Read the model definition and answer for the solid it produces. Units are mm, in the model's axes. A direction names the side the tool comes from. Coordinates: 2 decimals unless noted, no trailing zeros. Loops run counter-clockwise (first coordinate to the right, second up) from the corner with the lowest first, then second, coordinate; pieces in that order, holes last.
from build123d import *

# Parameters (mm, degrees)
F1_DEPTH = 76.2
F2_DEPTH = 211.582
F3_R     = 6.35
F4_DEPTH = 296.926


with BuildPart() as f1:
    # F0 (on Front) → F1 (new body)
    with BuildSketch(Plane.XZ):
        with BuildLine():
            Line((-75.994186, -26.958708), (-75.994186, -65.058708))
            Line((-75.994186, -65.058708), (0.205814, -65.058708))
            Line((0.205814, -65.058708), (0.205814, -26.958708))
            Line((0.205814, -26.958708), (41.952003, 20.148002))
            ThreePointArc((41.952003, 20.148002), (37.907157, 19.552642), (36.629202, 23.436206))
            Line((36.629202, 23.436206), (-37.894186, -26.958708))
            Line((-37.894186, -26.958708), (-110.240799, 29.427088))
            ThreePointArc((-110.240799, 29.427088), (-109.339718, 28.31636), (-109.017566, 26.922845))
            ThreePointArc((-109.017566, 26.922845), (-110.631205, 24.158288), (-113.831913, 24.203807))
            Line((-113.831913, 24.203807), (-75.994186, -26.958708))
        make_face()
        with BuildLine():
            ThreePointArc((36.629202, 23.436206), (37.907157, 19.552642), (41.952003, 20.148002))
            ThreePointArc((41.952003, 20.148002), (42.544402, 21.127687), (42.750814, 22.253792))
            ThreePointArc((42.750814, 22.253792), (41.820878, 24.498856), (39.575814, 25.428792))
            Line((39.575814, 25.428792), (36.629202, 23.436206))
        make_face()
        with BuildLine():
            ThreePointArc((-110.240799, 29.427088), (-114.808874, 28.721611), (-113.831913, 24.203807))
            ThreePointArc((-113.831913, 24.203807), (-110.631205, 24.158288), (-109.017566, 26.922845))
            ThreePointArc((-109.017566, 26.922845), (-109.339718, 28.31636), (-110.240799, 29.427088))
        make_face()
    extrude(amount=F1_DEPTH)

    # F1_face (on face) → F2 (cut)
    with BuildSketch(Plane(origin=(-38.414118, 0, -27.709483), x_dir=(1, 0, 0), z_dir=(0, 1, 0))):
        with BuildLine():
            Line((-37.580068, 37.349226), (-37.580068, -0.750774))
            Line((-37.580068, -0.750774), (-75.417795, -51.91329))
            ThreePointArc((-75.417795, -51.91329), (-76.394756, -56.431093), (-71.826681, -57.13657))
            Line((-71.826681, -57.13657), (0.519932, -0.750774))
            Line((0.519932, -0.750774), (77.989932, -53.138274))
            ThreePointArc((77.989932, -53.138274), (80.234996, -52.208338), (81.164932, -49.963274))
            ThreePointArc((81.164932, -49.963274), (80.958519, -48.837169), (80.366121, -47.857484))
            Line((80.366121, -47.857484), (38.619932, -0.750774))
            Line((38.619932, -0.750774), (38.619932, 37.349226))
            Line((38.619932, 37.349226), (-37.580068, 37.349226))
        make_face()
    extrude(amount=F2_DEPTH, mode=Mode.SUBTRACT)

    # F3 (on face) → F4 (cut)
    with BuildSketch(Plane.YZ.offset(0.205814)):
        with Locations((-38.1, -46.008708)):
            Circle(F3_R)
    extrude(amount=-F4_DEPTH, mode=Mode.SUBTRACT)


solid = f1.part
Q1. A cutting plane is placed at C-C (y = -58). Give the vertices of the cut face in (x, z) (3 decimals).
Findings below:
outline: (-113.832, 24.204) - (-75.994, -26.959) - (-75.994, -65.059) - (0.206, -65.059) - (0.206, -26.959) - (41.952, 20.148) arc R3.175 ccw to (42.751, 22.254) arc R3.175 ccw to (39.576, 25.429) - (-37.894, -26.959) - (-110.241, 29.427) arc R3.175 ccw (long way) to start
Q2. A cutting plane is placed at B-B (z = -7.5). Give the vertices of the cut face in (x, y).
Findings below:
outline: (-90.39, -76.2) - (-62.86, -76.2) - (-62.86, 0) - (-90.39, 0) - close; (-9.12, -76.2) - (17.45, -76.2) - (17.45, 0) - (-9.12, 0) - close
Q3. Determine the mould class of faces 4 (the face through (-37.361, -32.234, -48.441)), 5 (the face through (-37, -76.2, -27)), 6 (the face through (20.787, -37.567, -3.735)) for opening direction Y: +Y half, -Y half, draft (parallel to the pull), parting line (faces both ways), or undercut.
Findings below:
face 4: undercut
face 5: -Y half
face 6: draft
Q4. A cutting plane is placed at A-A (y = -38.1). Give the vertices of the cut face in (x, z) (3 decimals).
Findings below:
outline: (-113.832, 24.204) - (-75.994, -26.959) - (-75.994, -39.659) - (0.206, -39.659) - (0.206, -26.959) - (41.952, 20.148) arc R3.175 ccw to (42.751, 22.254) arc R3.175 ccw to (39.576, 25.429) - (-37.894, -26.959) - (-110.241, 29.427) arc R3.175 ccw (long way) to start; (-75.994, -65.059) - (0.206, -65.059) - (0.206, -52.359) - (-75.994, -52.359) - close
Q5. Which of the six approach directions +Z, -Z, +X, -X, +Y, -Y give full straight-line access (tool end or side, diameter ignored) to faces 1 (the face through (-75.994, -46, -46)), 2 (the face through (0.206, -38, -55)), 3 (the face through (-73.56, -37.57, 0.84))?
Findings below:
face 1: -Z, -X, +Y, -Y
face 2: -Z, +X, +Y, -Y
face 3: +Z, +Y, -Y
Q6. Flat-ended cylindrical pins translate along their axes: pin 1 Ø3 at (x, y) = (12, -43.5) entering from +Z; pin 2 Ø8 at (x, z) = (-98, 14) entering from +Y; pin 3 Ø19 at (y, z) = (-32, -39.5) entering from -X; pin 4 Ø1 at (x, y) = (-81, -30) entering from +Z. Find the tip coordinate at first contact, or state that the pin passes through.
Findings below:
pin 1: stops at z = 7.8
pin 2: stops at y = 0
pin 3: stops at x = -75.99
pin 4: stops at z = 7.03
Q7. Straight lines are drawn through the part: probe 1 along X at (y, z) = (-72, -45); probe 2 along Z at (x, y) = (-56, -38.1); probe 3 along Z at (x, y) = (-32, -38.1). For each, find the intervals that lie inside material, in ascending order.
Findings below:
probe 1: x = -75.99 to 0.21
probe 2: z = -65.06 to -52.36, -39.66 to -12.85
probe 3: z = -65.06 to -52.36, -39.66 to -22.97
Q8. A cutting plane is placed at D-D (x = -18.5). Give the vertices of the cut face in (y, z), then the cut area to 3 significant figures.
Findings below:
outline: (-76.2, -65.06) - (0, -65.06) - (0, -13.84) - (-76.2, -13.84) - close; hole circle Ø12.7 at (-38.1, -46.01)
area: 3,780 mm2
